```python
from build123d import *

# Parameters (mm, degrees)
F1_DEPTH = 300
F2_DEPTH = 300
F3_W     = 400
F3_H     = 300
F4_DEPTH = 22


with BuildPart() as f1:
    # F0 (on Front) → F1 (new body)
    with BuildSketch(Plane.XZ):
        Polygon((-150, 200), (-150, 0), (150, 0), (150, 200), (0, 200), align=None)
    extrude(amount=F1_DEPTH)

    # F0 (on Front) → F2 (join)
    with BuildSketch(Plane.XZ):
        Polygon((-150, 200), (-150, 0), (150, 0), (150, 200), (0, 200), align=None)
        Polygon((0, 300), (-150, 200), (0, 200), align=None)
        Polygon((0, 200), (150, 200), (0, 300), align=None)
    extrude(amount=F2_DEPTH)

    # F3 (on Top) → F4 (join)
    with BuildSketch(Plane.XY):
        with Locations((-5.947308, -152.311442)):
            Rectangle(F3_W, F3_H)
    extrude(amount=-F4_DEPTH)


solid = f1.part
```
Build history of the part. All positions in model axes, mm. A direction names the side the tool comes from. Give positions to 0.01 mm unless a question says otherwise; leave off trailing zeros. Loops run counter-clockwise (first coordinate to the right, second up) from the corner with the lowest first, then second, coordinate; pieces in that order, holes last. Notation, with made-up numbers: (-33, 3) -> (26, 3) arc R30 ccw to (26, 33) -> close; hole circle Ø2 at (4.25, -24). An arc over 180 degrees is marked (long way). One line per question, with ' | ' between items. Start each with the question number.
1) Cut at C-C (z = 254). Give the cut face in (x, y).
2) 3-axis set-ups, long thin cutter, end or side, ignore diameter. For faces 1 (the flat face through (-9, -2.311, -11)), 2 (the flat face through (150, -148, 99)), 3 (the flat face through (-2, -300, 119)): which of +Z, -Z, +X, -X, +Y, -Y reach the whole face in a straight line?
3) Pin check, flat tips, straight feed: pin 1 (10 mm diameter, centred on y = -72, z = 68, fed in from -X); pin 2 (6 mm diameter, centred on x = -120, z = 205, fed in from -Y); pin 3 (17.5 mm diameter, centred on x = -44.5, z = -16.5, fed in from +Y). Stop position of each tip, or through.
4) Cut at B-B (y = -105). Give the cut face in (x, z), plus the area to 3 significant figures.
5) Cut at D-D (x = -77). Give the cut face in (y, z).
6) Probe L1, parallel to Y at x = -37, z = 253; L2, parallel to X at y = -71, z = 9.5; L3, parallel to Z at x = -168.5, y = -58.5. List the from-to ranges inside material, lowest first.
7) Cut at A-A (x = -130). Give the cut face in (y, z).
Return value:
1) outline: (-69, -300) -> (69, -300) -> (69, 0) -> (-69, 0) -> close
2) face 1: -Z, +X, -X, +Y | face 2: +Z, +X, +Y, -Y | face 3: +Z, +X, -X, -Y
3) pin 1: x = -150 | pin 2: y = -300 | pin 3: y = -2.31
4) outline: (-205.95, -22) -> (194.05, -22) -> (194.05, 0) -> (150, 0) -> (150, 200) -> (0, 300) -> (-150, 200) -> (-150, 0) -> (-205.95, 0) -> close | area: 83,800 mm^2
5) outline: (-302.31, -22) -> (-2.31, -22) -> (-2.31, 0) -> (0, 0) -> (0, 248.67) -> (-300, 248.67) -> (-300, 0) -> (-302.31, 0) -> close
6) L1: -300 to 0 | L2: -150 to 150 | L3: -22 to 0
7) outline: (-302.31, -22) -> (-2.31, -22) -> (-2.31, 0) -> (0, 0) -> (0, 213.33) -> (-300, 213.33) -> (-300, 0) -> (-302.31, 0) -> close
